from build123d import *

# Parameters (mm, degrees)
SKETCH1_W                    = 38.1
SKETCH1_H                    = 25.4
BASE_FLANGE1_DEPTH           = 3.175
EDGE_FLANGE1_STRIP_W         = 14.1732
EDGE_FLANGE1_STRIP_H         = 3.175
EDGE_FLANGE1_STRIP_CUT_DEPTH = 25.4
EDGE_FLANGE1_DEPTH           = 25.4
SKETCH10_R                   = 3.175
CUT_EXTRUDE1_DEPTH           = 32.908355097


# Sheet-metal steps are written as plain solids
with BuildPart() as part:
    # Sketch1 → Base-Flange1 (new body)
    with BuildSketch(Plane(origin=(0, 0, 0), x_dir=(1, 0, 0), z_dir=(0, 1, 0))):
        Rectangle(SKETCH1_W, SKETCH1_H)
    extrude(amount=-BASE_FLANGE1_DEPTH)

    # Edge-Flange1 strip (across the edge) → Edge-Flange1 strip cut (cut)
    with BuildSketch(Plane(origin=(19.05, 0, 12.7), x_dir=(-1, 0, 0), z_dir=(0, 0, -1))):
        with Locations((-3.175, -1.5875)):
            Rectangle(EDGE_FLANGE1_STRIP_W, EDGE_FLANGE1_STRIP_H)
    extrude(amount=EDGE_FLANGE1_STRIP_CUT_DEPTH, mode=Mode.SUBTRACT)

    # Edge-Flange1 section (across the edge) → Edge-Flange1 (add)
    with BuildSketch(Plane(origin=(19.05, 0, 12.7), x_dir=(-1, 0, 0), z_dir=(0, 0, -1))):
        with BuildLine():
            Line((0, 0.7366), (0, 22.225))
            Line((0, 22.225), (3.175, 22.225))
            Line((3.175, 22.225), (3.175, 0.7366))
            ThreePointArc((3.175, 0.7366), (3.390745145, 0.215745145), (3.9116, 0))
            Line((3.9116, 0), (3.9116, -3.175))
            ThreePointArc((3.9116, -3.175), (1.145681115, -2.029318885), (0, 0.7366))
        make_face()
    extrude(amount=EDGE_FLANGE1_DEPTH)

    # Sketch10 → Cut-Extrude1 (cut, through all)
    with BuildSketch(Plane(origin=(0, 0, 0), x_dir=(1, 0, 0), z_dir=(0, 1, 0))):
        with Locations(Location((-6.35, 0, 0), (0, 0, 270))):
            Circle(SKETCH10_R)
    extrude(amount=-CUT_EXTRUDE1_DEPTH, mode=Mode.SUBTRACT)


solid = part.part
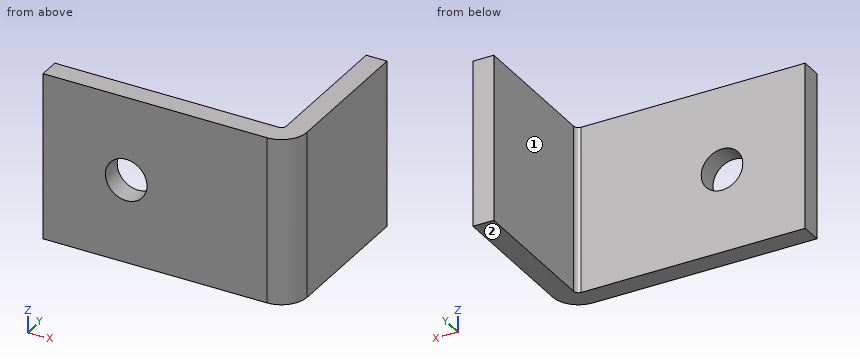
Input: part model. Units: mm. Frame: model coordinates. Face numbers are marked on the shaded views. A direction names the side the tool comes from. Give positions to 0.01 mm unless a question says otherwise; leave off trailing zeros. Order: outer loops, then holes, each group sorted by start corner. A loop starts at its lowest first (then second) coordinate and runs counter-clockwise, first axis right, second up. Notation, with made-up numbers: (85, 43.25) -> (135, 43.25) arc R19 ccw to (135, 70.25) -> close; hole circle Ø10 at (75.5, 34.25). An arc over 180 degrees is marked (long way). Use one line per item in the form item = value.
1) Section A-A, the plane x = -6.35. Return loops of the section in (y, z) (3 decimals).
Response values:
outline = (-3.175, -12.7) -> (0, -12.7) -> (0, -3.175) -> (-3.175, -3.175) -> close; (-3.175, 3.175) -> (0, 3.175) -> (0, 12.7) -> (-3.175, 12.7) -> close
2) Reachability of the marked faces 1 and 2 from +Z, -Z, +X, -X, +Y, -Y: full face, straight path, thin tool, end or side. Return the list, or none.
Response values:
face_1 = +Z, -Z, -X, +Y
face_2 = -Z, +X, -X, +Y, -Y
3) First-contact query: pin 1 Ø6 at (x, z) = (10, -4) entering from +Y. Flat tip, straight axial feed; report the tip coordinate or a pass-through.
Response values:
pin_1 = 0
4) Section B-B, the plane z = 0. Return loops of the section in (x, y) (3 decimals).
Response values:
outline = (-19.05, -3.175) -> (-9.525, -3.175) -> (-9.525, 0) -> (-19.05, 0) -> close; (-3.175, -3.175) -> (15.138, -3.175) arc R3.912 ccw to (19.05, 0.737) -> (19.05, 22.225) -> (15.875, 22.225) -> (15.875, 0.737) arc R0.737 cw to (15.138, 0) -> (-3.175, 0) -> close
5) Line query: probe 1 along Y at (x, z) = (-9.5, 8) (3 decimals); probe 2 along X at (y, z) = (-1.3, 0) (3 decimals); probe 3 along X at (y, z) = (11.25, -8) (3 decimals). Output: solid intervals per line, ascending.
Response values:
probe_1 = -3.175 to 0
probe_2 = -19.05 to -9.525, -3.175 to 18.478
probe_3 = 15.875 to 19.05
6) Section C-C, the plane z = 8.25. Return loops of the section in (x, y) (3 decimals), and give its area (3 significant figures).
Response values:
outline = (-19.05, -3.175) -> (15.138, -3.175) arc R3.912 ccw to (19.05, 0.737) -> (19.05, 22.225) -> (15.875, 22.225) -> (15.875, 0.737) arc R0.737 cw to (15.138, 0) -> (-19.05, 0) -> close
area = 188 mm^2
7) Section D-D, the plane y = -1.5. Return loops of the section in (x, z) (3 decimals).
Response values:
outline = (-19.05, -12.7) -> (18.347, -12.7) -> (18.347, 12.7) -> (-19.05, 12.7) -> close; hole circle Ø6.35 at (-6.35, 0)
